from build123d import *
from build123d.topology import SkipClean

# Parameters (mm, degrees)
EXTRUDE_2_DEPTH   = 4
SKETCH_1_R        = 5
EXTRUDE_2_2_DEPTH = 4
EXTRUDE_2_3_DEPTH = 4
SKETCH_1_4_R      = 7
SKETCH_1_4_R_2    = 5
EXTRUDE_3_DEPTH   = 14
EXTRUDE_START     = 10
EXTRUDE_4_DEPTH   = 10


with BuildPart() as part:
    # Sketch 1 → Extrude 2 (new body)
    with BuildSketch(Plane.XY):
        with BuildLine():
            ThreePointArc((-46.592863908, 7), (-39.592863908, 0), (-46.592863908, -7))
            Line((-46.592863908, -7), (113.407136092, -7))
            ThreePointArc((113.407136092, -7), (106.407136092, 0), (113.407136092, 7))
            Line((113.407136092, 7), (-46.592863908, 7))
        make_face()
    extrude(amount=EXTRUDE_2_DEPTH)



with BuildPart() as body_2:
    # Sketch 1 → Extrude 2 2 (new body)
    with BuildSketch(Plane.XY):
        with Locations((-46.592863908, 0)):
            Circle(SKETCH_1_R)
    extrude(amount=EXTRUDE_2_2_DEPTH)


with BuildPart() as body_3:
    # Sketch 1 → Extrude 2 3 (new body)
    with BuildSketch(Plane.XY):
        with Locations((113.407136092, 0)):
            Circle(SKETCH_1_R)
    extrude(amount=EXTRUDE_2_3_DEPTH)


with BuildPart() as part_1:
    add(part.part)

    add(body_2.part)  # Extrude 3 merges body 2

    add(body_3.part)  # Extrude 3 merges body 3
    # Sketch 1_4 → Extrude 3 (add)
    # profile 1 of 2: a face of its own
    with BuildSketch(Plane.XY):
        with Locations(Location((-46.592863908, 0, 0), (0, 0, 270))):
            Circle(SKETCH_1_4_R)
        with Locations((-46.592863908, 0)):
            Circle(SKETCH_1_4_R_2, mode=Mode.SUBTRACT)
    # profile 2 of 2: a face of its own
    with BuildSketch(Plane.XY):
        with Locations(Location((113.407136092, 0, 0), (0, 0, 270))):
            Circle(SKETCH_1_4_R)
        with Locations((113.407136092, 0)):
            Circle(SKETCH_1_4_R_2, mode=Mode.SUBTRACT)
    extrude(amount=EXTRUDE_3_DEPTH)

    # Sketch 2 → Extrude 4 (add)
    with SkipClean():  # the faces are left unmerged after this step: merging them gives an invalid solid
        with BuildSketch(Plane(origin=(0, 0, 0), x_dir=(-1, 0, 0), z_dir=(0, 0, -1)).offset(EXTRUDE_START)):
            with BuildLine():
                Line((46.592863908, 7), (-113.407136092, 7))
                ThreePointArc((-113.407136092, 7), (-120.407136092, 0), (-113.407136092, -7))
                Line((-113.407136092, -7), (46.592863908, -7))
                ThreePointArc((46.592863908, -7), (53.592863908, 0), (46.592863908, 7))
            make_face()
        extrude(amount=-EXTRUDE_4_DEPTH)


solid = part_1.part
Design review of the part built by this model. Coordinates are the model's own, in mm. A direction names the side the tool comes from. Coordinates: 2 decimals unless noted, no trailing zeros. Write each loop counter-clockwise with the first axis right and the second up, starting at its lowest first coordinate (ties: lowest second). Pieces come first, ordered by that corner, then holes. Notation, with made-up numbers: (55, 43) -> (80, 43) arc R22 ccw to (80, 81) -> close; hole circle Ø10 at (42, 82.25). An arc over 180 degrees is marked (long way). Write each question's results on one line, items separated by ' | '. Start each with the question number.
(1) For line 1 along Z through (x, y) = (16, -3.75); line 2 along X through (y, z) = (-2, 1.25); line 3 along X through (y, z) = (5.25, 3), list the stretches that pass through material, from the lowest coordinate up. Write a range as from..to.
(2) Tool access review of faces 4 (the face through (-41.974, -1.915, 8.93)), 5 (the face through (-45, 5, 14)): name each direction out of +Z, -Z, +X, -X, +Y, -Y from which nothing blocks a thin tool from reaching the whole face with its end or side.
(3) Take a section at C-C on x = -26. Write out the cut boundary in (y, z).
(4) Take a section at A-A on y = 0. Write out the cut boundary in (x, z), and give its area (3 significant figures).
(5) Clearance check with flat-ended pins moving along their axes: P1, Ø1.5, axis at y = 2, z = 9, coming from the -X side; P2, Ø7, axis at x = 0.5, y = -1, coming from the +Z side. State where each tip first meets the part, or that it passes through.
(6) The part is to be moulded in two halves that separate along Y. For faces 1 (the face through (108.41, 0.22, 8.93)), 2 (the face through (35, 0, -10)), 3 (the face through (32, 7, -3)), say which applies: pulls with the +Y half, pulls with the -Y half, needs draft (parallel to the pull), parting line crosses it, or undercut.
(7) Take a section at B-B on z = -5.5. Write out the cut boundary in (x, y).
Results found:
1) line 1: z = -10..4 | line 2: x = -53.3..120.12 | line 3: x = -51.22..118.04
2) face 4: +Z | face 5: +Z, +X, -X, +Y, -Y
3) outline: (-7, -10) -> (7, -10) -> (7, 4) -> (-7, 4) -> close
4) outline: (-53.59, -10) -> (120.41, -10) -> (120.41, 14) -> (118.41, 14) -> (118.41, 4) -> (108.41, 4) -> (108.41, 14) -> (106.41, 14) -> (106.41, 4) -> (-39.59, 4) -> (-39.59, 14) -> (-41.59, 14) -> (-41.59, 4) -> (-51.59, 4) -> (-51.59, 14) -> (-53.59, 14) -> close | area: 2,520 mm2
5) P1: stops at x = -53.48 | P2: stops at z = 4
6) face 1: undercut | face 2: needs draft | face 3: pulls with the +Y half
7) outline: (-46.59, -7) -> (113.41, -7) arc R7 ccw to (113.41, 7) -> (-46.59, 7) arc R7 ccw to start
